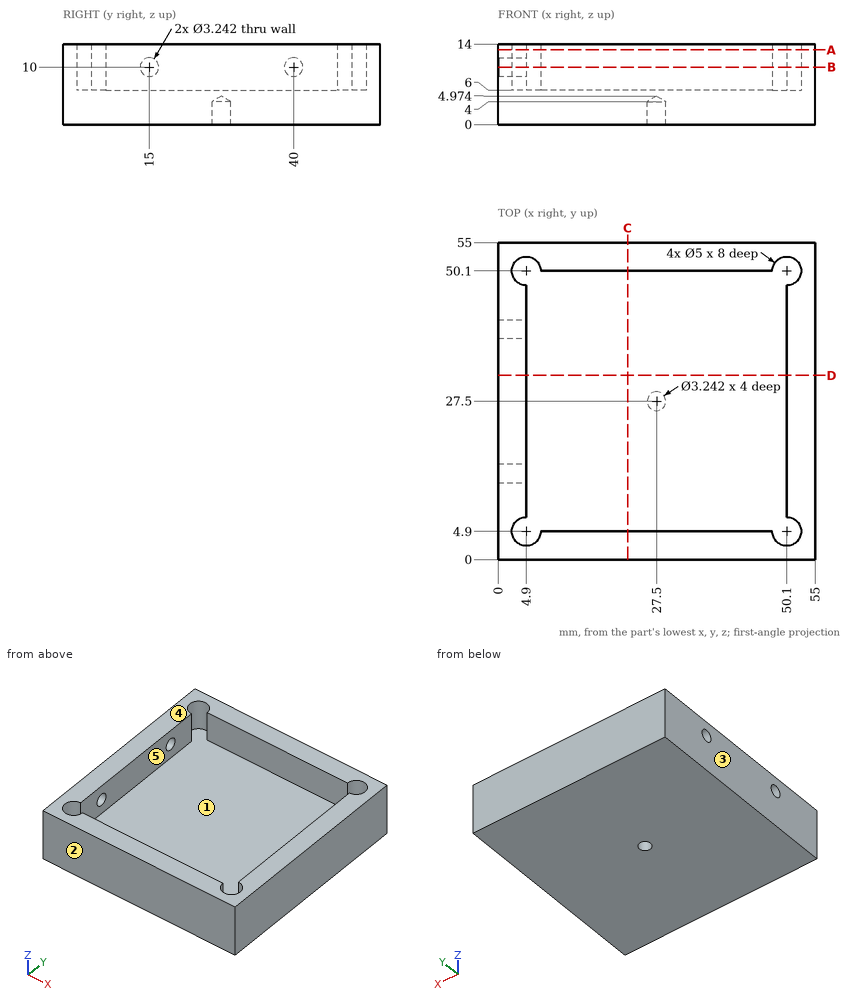
For this review, use the dimensioned drawing (mm, ordinates from the lowest corner) and the shaded views. A direction names the side the tool comes from. Coordinates: 2 decimals unless noted, no trailing zeros. Order: outer loops, then holes, each group sorted by start corner. A loop starts at its lowest first (then second) coordinate and runs counter-clockwise, first axis right, second up. Notation, with made-up numbers: (75, 85) - (95, 85) arc R8 ccw to (95, 97) - close; hole circle Ø2 at (61, 25). An arc over 180 degrees is marked (long way). Answer as a JSON object with one key per item and string values. Group by question number.
1. Clearance check with flat-ended pins moving along their axes: P1, Ø3, axis at y = 15, z = 10, coming from the -X side; P2, Ø3, axis at x = 50.1, y = 4.9, coming from the +Z side; P3, Ø2.5, axis at x = 27.5, y = 27.5, coming from the -Z side. State where each tip first meets the part, or that it passes through.
2. We need section A-A on z = 13. State the section outline as (x, y) points, then the cut area to 3 significant figures.
3. We need section B-B on z = 10. State the section outline as (x, y) points, then the cut area to 3 significant figures.
4. The part is to be moulded in two halves that separate along Y. For the marked faces 1, 2 and 3, say which applies: pulls with the +Y half, pulls with the -Y half, needs draft (parallel to the pull), parting line crosses it, or undercut.
5. For the marked faces 4 and 5, list the 3-axis set-ups (+Z, -Z, +X, -X, +Y, -Y) from which the entire face can be reached by the end or side of a thin tool; tool diameter is ignored.
6. We need section C-C on x = 22.5. State the section outline as (y, z) points.
7. For probe 1 along Y at (x, z) = (2.35, 10); probe 2 along X at (y, z) = (25.5, 6.25); probe 3 along Z at (x, y) = (1, 15), list the stretches that pass through material, from the lowest coordinate up.
Final values:
{
 "1": {"P1": "x = 50.1", "P2": "z = 6", "P3": "z = 4.22"},
 "2": {"outline": "(0, 0) - (55, 0) - (55, 55) - (0, 55) - close; hole (4.9, 7.4) arc R2.5 ccw (long way) to (7.4, 4.9) - (47.6, 4.9) arc R2.5 ccw (long way) to (50.1, 7.4) - (50.1, 47.6) arc R2.5 ccw (long way) to (47.6, 50.1) - (7.4, 50.1) arc R2.5 ccw (long way) to (4.9, 47.6) - close", "area": "923 mm²"},
 "3": {"outline": "(0, 0) - (55, 0) - (55, 55) - (0, 55) - (0, 41.62) - (4.9, 41.62) - (4.9, 47.6) arc R2.5 cw (long way) to (7.4, 50.1) - (47.6, 50.1) arc R2.5 cw (long way) to (50.1, 47.6) - (50.1, 7.4) arc R2.5 cw (long way) to (47.6, 4.9) - (7.4, 4.9) arc R2.5 cw (long way) to (4.9, 7.4) - (4.9, 13.38) - (0, 13.38) - close; (0, 16.62) - (4.9, 16.62) - (4.9, 38.38) - (0, 38.38) - close", "area": "891 mm²"},
 "4": {"face 1": "undercut", "face 2": "pulls with the -Y half", "face 3": "needs draft"},
 "5": {"face 4": "+Z, +X, -X, +Y, -Y", "face 5": "+Z"},
 "6": {"outline": "(0, 0) - (55, 0) - (55, 14) - (50.1, 14) - (50.1, 6) - (4.9, 6) - (4.9, 14) - (0, 14) - close"},
 "7": {"probe 1": "0 to 13.38, 16.62 to 38.38, 41.62 to 55", "probe 2": "0 to 4.9, 50.1 to 55", "probe 3": "0 to 8.38, 11.62 to 14"}
}
